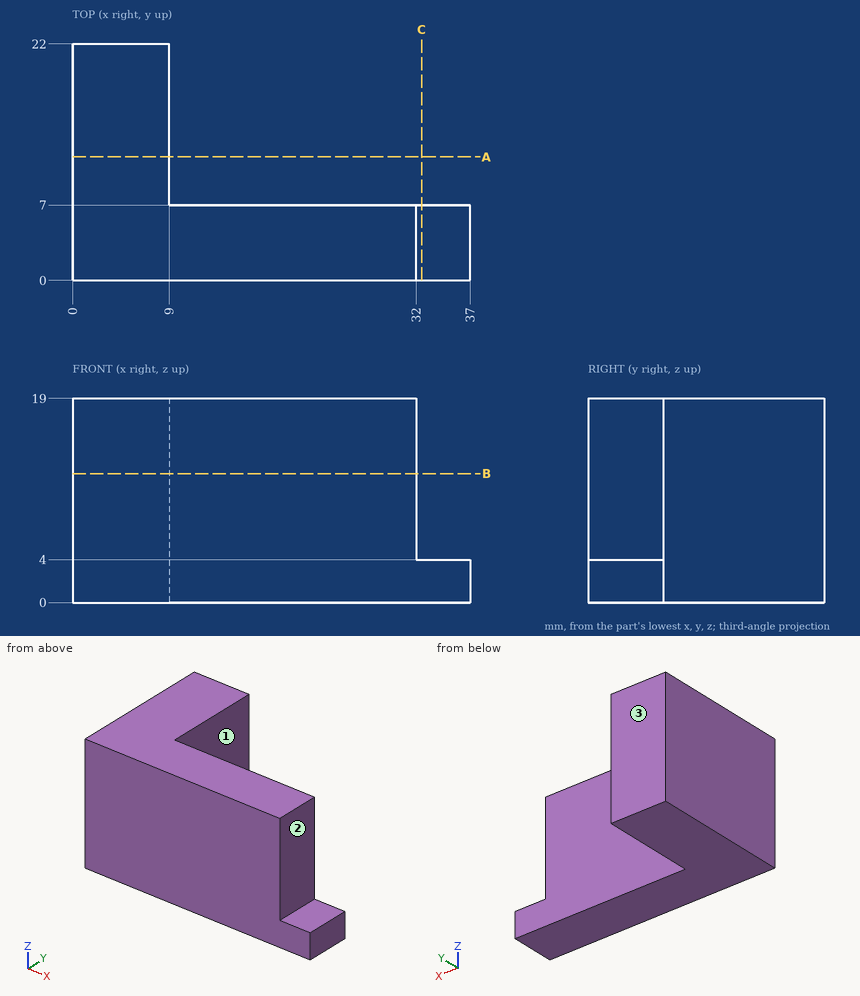
Verification items for this drawing (mm, ordinates from the low corner). A direction names the side the tool comes from. Coordinates: 2 decimals unless noted, no trailing zeros. Write each loop counter-clockwise with the first axis right and the second up, starting at its lowest first coordinate (ties: lowest second). Pieces come first, ordered by that corner, then holes. Notation, with made-up numbers: (8.25, 52.5) -> (12.25, 52.5) arc R33 ccw to (12.25, 83.5) -> close; hole circle Ø4 at (-29, 43). An arc over 180 degrees is marked (long way). Use CSV: the item, a comma, the result in double quotes. Start each with the question number.
Item 1: Cross-section at A-A, the plane y = 11.5. Record the cut outline in (x, z), plus the area to 3 significant figures.
Item 2: Depth check by flat-ended pin: pin 1 Ø5.5 at (y, z) = (4.5, 11.5) entering from +X; pin 2 Ø1 at (y, z) = (19, 10) entering from +X; pin 3 Ø4 at (x, y) = (34.5, 2) entering from +Z. Enter the tip coordinate at first touch or a pass-through.
Item 3: Cross-section at B-B, the plane z = 12. Record the cut outline in (x, y).
Item 4: Cross-section at C-C, the plane x = 32.5. Record the cut outline in (y, z), plus the area to 3 significant figures.
Item 5: Set-up check for the marked faces 1, 2 and 3: record each of +Z, -Z, +X, -X, +Y, -Y from which the full face is reachable in a straight line by a thin tool's end or side.
Item 6: Thickness scan on line 1 (Y direction, x = 25, z = 18); line 2 (X direction, y = 15.75, z = 10.75); line 3 (X direction, y = 3.75, z = 5). Record the ranges inside material, lowest first.
Answers:
1,outline,"(0, 0) -> (9, 0) -> (9, 19) -> (0, 19) -> close"
1,area,"171 mm^2"
2,pin 1,"x = 32"
2,pin 2,"x = 9"
2,pin 3,"z = 4"
3,outline,"(0, 0) -> (32, 0) -> (32, 7) -> (9, 7) -> (9, 22) -> (0, 22) -> close"
4,outline,"(0, 0) -> (7, 0) -> (7, 4) -> (0, 4) -> close"
4,area,"28.0 mm^2"
5,face 1,"+Z, -Z, +X, +Y"
5,face 2,"+Z, +X, +Y, -Y"
5,face 3,"+Z, -Z, +X, -X, +Y"
6,line 1,"0 to 7"
6,line 2,"0 to 9"
6,line 3,"0 to 32"
